Here's how the part is built. I have some questions about the finished solid (model axes, mm). A direction names the side the tool comes from. Give positions to 0.01 mm unless a question says otherwise; leave off trailing zeros. Loops run counter-clockwise (first coordinate to the right, second up) from the corner with the lowest first, then second, coordinate; pieces in that order, holes last.
Q1. Suppose I cut it at D-D (z = 0). List the corners of the cut face in (x, y) for me.
Q2. Suppose I cut it at C-C (y = 5). List the corners of the cut face in (x, z) for me, and give its area (3 significant figures).
Q3. Suppose I cut it at A-A (x = 0). List the corners of the cut face in (y, z) for me, and give its area (3 significant figures).
Q4. For faces 4 (the face through (0.364, -8.532, -8.272)), 5 (the face through (3, -13.4, 6)), 6 (the face through (4.66, 10.12, -5.09)), which set-ups out of +Z, -Z, +X, -X, +Y, -Y let a thin tool reach every point of the face, with its end or its side?
Q5. I'm going to push flat-ended pins straight in: P1, Ø6, axis at x = -5.5, y = 11, coming from the -Z side; P2, Ø9, axis at x = 0, y = -9.4, coming from the -Z side; P3, Ø4, axis at x = 7, y = 13, coming from the +Z side. Where does each tip first touch, or does it pass through?
Q6. Thinking about a two-plate mould opening in X: for faces 1 (the face through (0.276, -8.532, -6.274)), 2 (the face through (6.015, 10.12, -6.56)), 3 (the face through (6, -17.8, 3)), which applies, pulls with the +X half, pulls with the -X half, needs draft (parallel to the pull), parting line crosses it, or undercut?
Q7. Suppose I cut it at B-B (z = 5). List the corners of the cut face in (x, y) for me (3 decimals), and give its area (3 significant figures).
Q8. I need wall thicknesses on probe 1 along Y at (x, z) = (0, 6.7); probe 2 along Y at (x, z) = (0, 7.05); probe 3 along X at (y, z) = (7.5, 0). Which ranges of each line are inside material? Lowest first, please.
```python
from build123d import *

# Parameters (mm, degrees)
BOSS_EXTRUDE1_DEPTH      = 1
BOSS_EXTRUDE1_DEPTH_BACK = 17.8
SKETCH1_R                = 8.28
SKETCH1_R_2              = 6.28
SKETCH2_R                = 8.9
SKETCH2_R_2              = 6.9
BOSS_EXTRUDE2_DEPTH      = 18.5
SKETCH3_R                = 5
CUT_EXTRUDE1_DEPTH       = 24.209265391


with BuildPart() as part:
    # Sketch1 → Boss-Extrude1 (new, two sides: drawn at the far end of the back side and taken through both)
    with BuildSketch(Plane(origin=(0, 0, 0), x_dir=(1, 0, 0), z_dir=(0, 1, 0)).offset(-BOSS_EXTRUDE1_DEPTH_BACK)):
        with Locations(Location((0, 0, 0), (0, 0, 270))):
            Circle(SKETCH1_R)
        with Locations(Location((0, 0, 0), (0, 0, 270))):
            Circle(SKETCH1_R_2, mode=Mode.SUBTRACT)
    extrude(amount=BOSS_EXTRUDE1_DEPTH + BOSS_EXTRUDE1_DEPTH_BACK)

    # Sketch2 → Boss-Extrude2 (add)
    with BuildSketch(Plane(origin=(0, 1, 0), x_dir=(1, 0, 0), z_dir=(0, 1, 0))):
        with Locations(Location((0, 0, 0), (0, 0, 270))):
            Circle(SKETCH2_R)
        with Locations(Location((0, 0, 0), (0, 0, 270))):
            Circle(SKETCH2_R_2, mode=Mode.SUBTRACT)
    extrude(amount=BOSS_EXTRUDE2_DEPTH)

    # Sketch3 → Cut-Extrude1 (cut, through all)
    with BuildSketch(Plane.XY):
        with Locations(Location((0, -9.4, 0), (0, 0, 90.000000004))):
            Circle(SKETCH3_R)
    extrude(amount=CUT_EXTRUDE1_DEPTH, mode=Mode.SUBTRACT)


solid = part.part
```
Solutions:
1. outline: (-8.9, 1) - (-8.28, 1) - (-8.28, -17.8) - (-6.28, -17.8) - (-6.28, 1) - (-6.9, 1) - (-6.9, 19.5) - (-8.9, 19.5) - close; (6.28, -17.8) - (8.28, -17.8) - (8.28, 1) - (8.9, 1) - (8.9, 19.5) - (6.9, 19.5) - (6.9, 1) - (6.28, 1) - close
2. outline: circle Ø17.8 at (0, 0); hole circle Ø13.8 at (0, 0)
2. area: 99.3 mm2
3. outline: (-17.8, -8.28) - (1, -8.28) - (1, -8.9) - (19.5, -8.9) - (19.5, -6.9) - (1, -6.9) - (1, -6.28) - (-17.8, -6.28) - close; (-17.8, 6.28) - (-14.4, 6.28) - (-14.4, 8.28) - (-17.8, 8.28) - close; (-4.4, 6.28) - (1, 6.28) - (1, 6.9) - (19.5, 6.9) - (19.5, 8.9) - (1, 8.9) - (1, 8.28) - (-4.4, 8.28) - close
3. area: 129 mm2
4. face 4: -Y
4. face 5: +Z
4. face 6: +Y
5. P1: stops at z = -8.54
5. P2: stops at z = -8.28
5. P3: stops at z = 7.36
6. face 1: undercut
6. face 2: parting line crosses it
6. face 3: needs draft
7. outline: (-7.363, 1) - (-6.6, 1) - (-6.6, -17.8) - (-3.8, -17.8) - (-3.8, -12.65) arc R5 cw to (-3.8, -6.15) - (-3.8, 1) - (-4.755, 1) - (-4.755, 19.5) - (-7.363, 19.5) - close; (3.8, -17.8) - (6.6, -17.8) - (6.6, 1) - (7.363, 1) - (7.363, 19.5) - (4.755, 19.5) - (4.755, 1) - (3.8, 1) - (3.8, -6.15) arc R5 cw to (3.8, -12.65) - close
7. area: 191 mm2
8. probe 1: y = -17.8 to -14.4, -4.4 to 1
8. probe 2: y = -17.8 to -14.4, -4.4 to 19.5
8. probe 3: x = -8.9 to -6.9, 6.9 to 8.9
